Drawing for the job (mm, zero at the part's lowest x, y, z). Coordinates: 2 decimals unless noted, no trailing zeros. Write each loop counter-clockwise with the first axis right and the second up, starting at its lowest first coordinate (ties: lowest second). Pieces come first, ordered by that corner, then holes. Notation, with made-up numbers: (41, 82.25) -> (93, 82.25) arc R9 cw to (93, 92.25) -> close; hole circle Ø6 at (18, 65). An arc over 180 degrees is marked (long way). Answer as CSV lines item,"result".
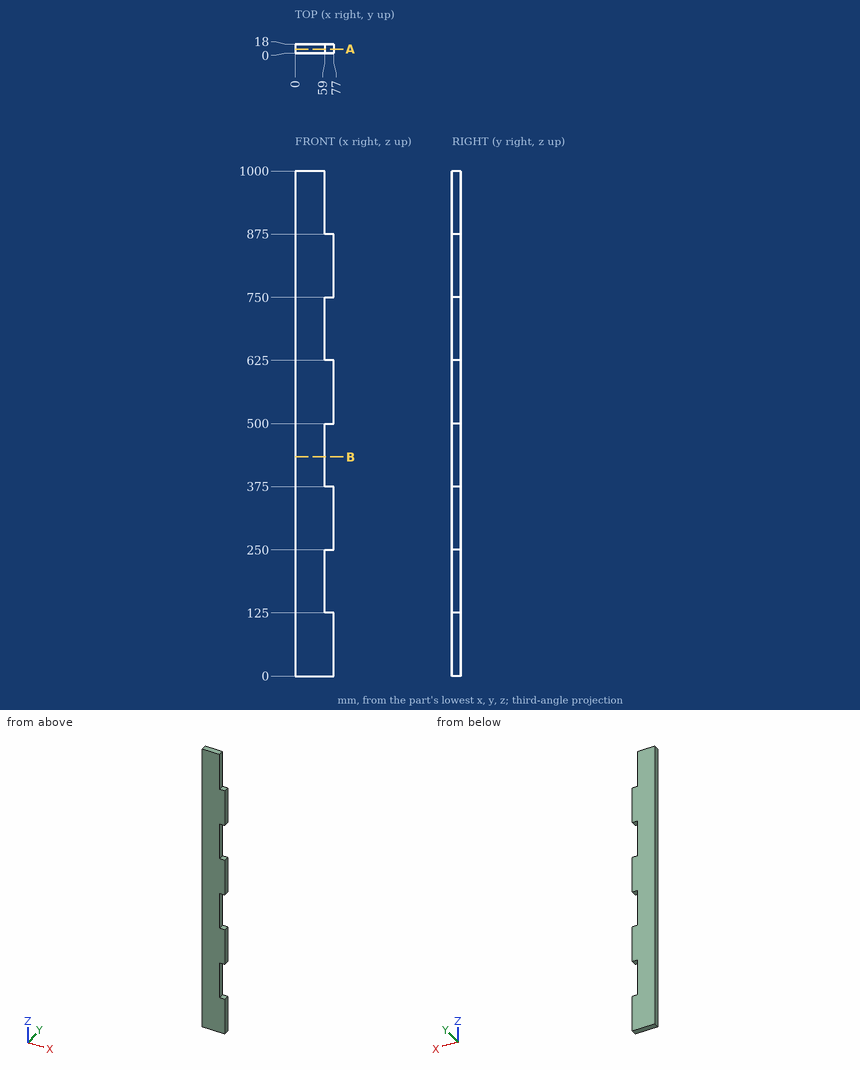
Item 1: Saw through at B-B on z = 434. Give the cut face in (x, y), and give its area (3 significant figures).
Answer below:
outline,"(0, 0) -> (59, 0) -> (59, 18) -> (0, 18) -> close"
area,"1,060 mm2"
Item 2: Saw through at A-A on y = 8. Give the cut face in (x, z), and give its area (3 significant figures).
Answer below:
outline,"(0, 0) -> (77, 0) -> (77, 125) -> (59, 125) -> (59, 250) -> (77, 250) -> (77, 375) -> (59, 375) -> (59, 500) -> (77, 500) -> (77, 625) -> (59, 625) -> (59, 750) -> (77, 750) -> (77, 875) -> (59, 875) -> (59, 1000) -> (0, 1000) -> close"
area,"68,000 mm2"
Item 3: Flat gauge pins, fed straight in: pin 1 (9 mm diameter, centred on y = 13, z = 667, fed in from +X); pin 2 (5 mm diameter, centred on x = 38, y = 10, fed in from -Z); pin 3 (9 mm diameter, centred on x = 71.5, y = 9, fed in from +Z). Where does each tip first touch, or does it go through?
Answer below:
pin 1,"stops at x = 59"
pin 2,"stops at z = 0"
pin 3,"stops at z = 875"
Item 4: Wall check: line 1 (Z direction, x = 61, y = 7.75); line 2 (X direction, y = 11, z = 639.5). Give the ranges that are in metal, low to high. Write a range as from..to.
Answer below:
line 1,"z = 0..125, 250..375, 500..625, 750..875"
line 2,"x = 0..59"
